For this review, take the finished solid that the model builds, in its own axes (mm). Coordinates: 2 decimals unless noted, no trailing zeros.
```python
from build123d import *

# Parameters (mm, degrees)
SKETCH1_W           = 408.5
SKETCH1_H           = 122.3
SKETCH1_R           = 1.75
SKETCH1_W_2         = 16
SKETCH1_H_2         = 7.15
SKETCH1_W_3         = 11.25
SKETCH1_H_3         = 8
SKETCH1_W_4         = 15
BOSS_EXTRUDE1_DEPTH = 2


with BuildPart() as part:
    # Sketch1 → Boss-Extrude1 (new body)
    with BuildSketch(Plane(origin=(0, 0, 0), x_dir=(1, 0, 0), z_dir=(0, 1, 0))):
        with Locations((204.25, 61.15)):
            Rectangle(SKETCH1_W, SKETCH1_H)
        with Locations(Location((39, 72.3, 0), (0, 0, 270))):
            Circle(SKETCH1_R, mode=Mode.SUBTRACT)
        with Locations(Location((69, 72.3, 0), (0, 0, 270))):
            Circle(SKETCH1_R, mode=Mode.SUBTRACT)
        with Locations((317.09, 16.875)):
            Rectangle(SKETCH1_W_2, SKETCH1_H_2, mode=Mode.SUBTRACT)
        with Locations((379.5, 17.3)):
            Rectangle(SKETCH1_W_3, SKETCH1_H_3, mode=Mode.SUBTRACT)
        with Locations((355.19, 16.875)):
            Rectangle(SKETCH1_W_2, SKETCH1_H_2, mode=Mode.SUBTRACT)
        with Locations((278.99, 16.875)):
            Rectangle(SKETCH1_W_2, SKETCH1_H_2, mode=Mode.SUBTRACT)
        with Locations((240.89, 16.875)):
            Rectangle(SKETCH1_W_2, SKETCH1_H_2, mode=Mode.SUBTRACT)
        with Locations((202.79, 16.875)):
            Rectangle(SKETCH1_W_2, SKETCH1_H_2, mode=Mode.SUBTRACT)
        with Locations((164.69, 16.875)):
            Rectangle(SKETCH1_W_2, SKETCH1_H_2, mode=Mode.SUBTRACT)
        with Locations((126.59, 16.875)):
            Rectangle(SKETCH1_W_2, SKETCH1_H_2, mode=Mode.SUBTRACT)
        with Locations((88.49, 16.875)):
            Rectangle(SKETCH1_W_2, SKETCH1_H_2, mode=Mode.SUBTRACT)
        with Locations((50.39, 16.875)):
            Rectangle(SKETCH1_W_2, SKETCH1_H_2, mode=Mode.SUBTRACT)
        with Locations((54, 72.3)):
            Rectangle(SKETCH1_W_4, SKETCH1_H_3, mode=Mode.SUBTRACT)
    extrude(amount=BOSS_EXTRUDE1_DEPTH)


solid = part.part
```
1) For L1, parallel to X at y = 0.2, z = -72; L2, parallel to Z at x = 92, y = 1.25; L3, parallel to Z at x = 385, y = 1.2, list the stretches that pass through material, from the lowest coordinate up.
2) Clearance check with flat-ended pins moving along their axes: P1, Ø8, axis at x = 98, z = -106.5, coming from the -Y side; P2, Ø3, axis at x = 69, z = -72.3, coming from the -Y side. State where each tip first meets the part, or that it passes through.
3) Consider section A-A (y = 1.35). Count the separate pieces of the cut face and the enclosed holes in it, then the cut area to 3 significant figures.
Results:
1. L1: x = 0 to 37.28, 40.72 to 46.5, 61.5 to 67.28, 70.72 to 408.5
1. L2: z = -122.3 to -20.45, -13.3 to 0
1. L3: z = -122.3 to -21.3, -13.3 to 0
2. P1: stops at y = 0
2. P2: passes through
3. separate pieces: 1
3. enclosed holes: 13
3. area: 48,700 mm2
